Build history of the part. All positions in model axes, mm. Face numbers are marked on the shaded views. A direction names the side the tool comes from. Give positions to 0.01 mm unless a question says otherwise; leave off trailing zeros. Write each loop counter-clockwise with the first axis right and the second up, starting at its lowest first coordinate (ties: lowest second). Pieces come first, ordered by that corner, then holes. Notation, with made-up numbers: (76, 85) -> (116, 85) arc R29 ccw to (116, 113) -> close; hole circle Ø8 at (-21.5, -29.75). An arc over 180 degrees is marked (long way). Put each result on its own line as item: value.
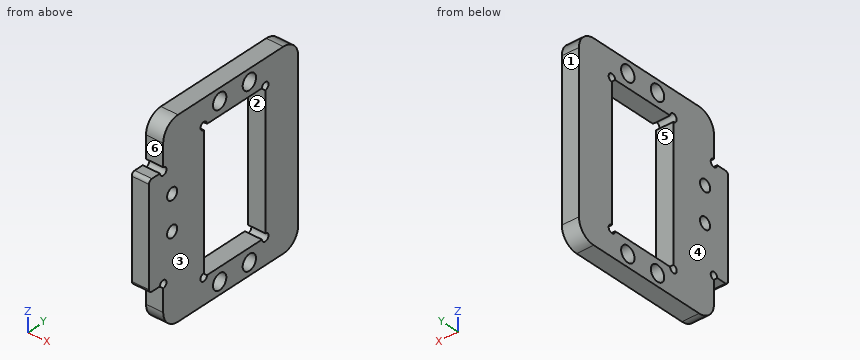
from build123d import *

# Parameters (mm, degrees)
SKETCH_1_W                   = 55
SKETCH_1_H                   = 45.45
SKETCH_1_W_2                 = 40.2
SKETCH_1_H_2                 = 20.7
EXTRUDE_1_DEPTH              = 5
SKETCH_2_W                   = 30
SKETCH_2_H                   = 4.8
EXTRUDE_2_DEPTH              = 5
FILLET_1_R                   = 5
SKETCH_3_R                   = 1.1
CUT_EXTRUDE_1_DEPTH          = 5
FILLET_2_R                   = 1
HOLE_WIZARD_M3_1_D           = 3.4
M4_CLEARANCE_HOLE1_OUTLINE_R = 2.25
M4_CLEARANCE_HOLE1_DEPTH     = 5


# Read off the part's stored shape, not the designer's step: M4 Clearance Hole1
with BuildPart() as part:
    # 草图1 → 凸台-拉伸1 (new body)
    with BuildSketch(Plane(origin=(0, 0, 0), x_dir=(0, 0, -1), z_dir=(1, 0, 0))):
        with Locations((27.5, 22.725)):
            Rectangle(SKETCH_1_W, SKETCH_1_H)
        with Locations((27.5, 24)):
            Rectangle(SKETCH_1_W_2, SKETCH_1_H_2, mode=Mode.SUBTRACT)
    extrude(amount=EXTRUDE_1_DEPTH)

    # 草图2 → 凸台-拉伸2 (add)
    with BuildSketch(Plane(origin=(5, 0, 0), x_dir=(0, 0, -1), z_dir=(1, 0, 0))):
        with Locations((27.5, -2.4)):
            Rectangle(SKETCH_2_W, SKETCH_2_H)
    extrude(amount=-EXTRUDE_2_DEPTH)

    # 圆角1
    fillet_1_edges = [part.edges().sort_by_distance(p)[0] for p in [
        (2.5, 45.45, 0),
        (2.5, 45.45, -55),
        (2.5, 0, -55),
        (2.5, 0, 0),
    ]]
    fillet(fillet_1_edges, radius=FILLET_1_R)

    # 草图3 → 切除-拉伸1 (cut)
    with BuildSketch(Plane(origin=(5, 0, 0), x_dir=(0, 0, -1), z_dir=(1, 0, 0))):
        with Locations((12.5, 0)):
            Circle(SKETCH_3_R)
        with Locations((42.5, 0)):
            Circle(SKETCH_3_R)
        with Locations((7.4, 13.65)):
            Circle(SKETCH_3_R)
        with Locations((7.4, 34.35)):
            Circle(SKETCH_3_R)
        with Locations((47.6, 34.35)):
            Circle(SKETCH_3_R)
        with Locations((47.6, 13.65)):
            Circle(SKETCH_3_R)
    extrude(amount=-CUT_EXTRUDE_1_DEPTH, mode=Mode.SUBTRACT)

    # 圆角2
    fillet_2_edges = [part.edges().sort_by_distance(p)[0] for p in [
        (2.5, -4.8, -42.5),
        (2.5, -4.8, -12.5),
    ]]
    fillet(fillet_2_edges, radius=FILLET_2_R)

    # M3 间隙孔1 (through all)
    with Locations(Plane.ZY):
        with Locations((-20, 3), (-30, 3)):
            Hole(HOLE_WIZARD_M3_1_D / 2)

    # M4 Clearance Hole1 outline → M4 Clearance Hole1 (cut)
    with BuildSketch(Plane.YZ):
        with Locations((29, -3.5)):
            Circle(M4_CLEARANCE_HOLE1_OUTLINE_R)
        with Locations((19, -51.5)):
            Circle(M4_CLEARANCE_HOLE1_OUTLINE_R)
        with Locations((19, -3.5)):
            Circle(M4_CLEARANCE_HOLE1_OUTLINE_R)
        with Locations((29, -51.5)):
            Circle(M4_CLEARANCE_HOLE1_OUTLINE_R)
    extrude(amount=M4_CLEARANCE_HOLE1_DEPTH, mode=Mode.SUBTRACT)


solid = part.part
1) Pin check, flat tips, straight feed: pin 1 (1.5 mm diameter, centred on x = 2, z = -48.5, fed in from -Y); pin 2 (1.8 mm diameter, centred on y = 0, z = -12.5, fed in from -X); pin 3 (2 mm diameter, centred on x = 2, y = -2.5, fed in from -Z). Stop position of each tip, or through.
Filled sheet:
pin 1: y = 0
pin 2: through
pin 3: z = -42.5
2) Slice it at C-C (x = 4.3). Give the number of separate pieces and of enclosed holes in the cut face, plus the area to 3 significant figures.
Filled sheet:
separate pieces: 1
enclosed holes: 7
area: 1,690 mm2
3) Slice it at D-D (y = 3). Write the cut outline in (x, z), plus the area to 3 significant figures.
Filled sheet:
outline: (0, -54.58) -> (5, -54.58) -> (5, -31.7) -> (0, -31.7) -> close; (0, -28.3) -> (5, -28.3) -> (5, -21.7) -> (0, -21.7) -> close; (0, -18.3) -> (5, -18.3) -> (5, -0.42) -> (0, -0.42) -> close
area: 237 mm2
4) Tool access for the marked faces 4, 5 and 6: list every direction of +Z, -Z, +X, -X, +Y, -Y with a clear straight run to the whole face (end or side of a thin tool).
Filled sheet:
face 4: +Z, -Z, -X, +Y, -Y
face 5: +X, -X
face 6: +Z, +X, -X, -Y
5) Wall check: L1, parallel to Y at x = 2.3, z = -30; L2, parallel to Z at x = 1, y = 23.5; L3, parallel to Y at x = 1.15, z = -32.5. Give the ranges that are in metal, low to high.
Filled sheet:
L1: -4.8 to 1.3, 4.7 to 13.65, 34.35 to 45.45
L2: -55 to -47.6, -7.4 to 0
L3: -4.8 to 13.65, 34.35 to 45.45
6) Slice it at B-B (y = 29). Write the cut outline in (x, z), plus the area to 3 significant figures.
Filled sheet:
outline: (0, -55) -> (5, -55) -> (5, -53.75) -> (0, -53.75) -> close; (0, -49.25) -> (5, -49.25) -> (5, -47.6) -> (0, -47.6) -> close; (0, -7.4) -> (5, -7.4) -> (5, -5.75) -> (0, -5.75) -> close; (0, -1.25) -> (5, -1.25) -> (5, 0) -> (0, 0) -> close
area: 29.0 mm2
7) Slice it at A-A (z = -23). Write the cut outline in (x, y).
Filled sheet:
outline: (0, -4.8) -> (5, -4.8) -> (5, 13.65) -> (0, 13.65) -> close; (0, 34.35) -> (5, 34.35) -> (5, 45.45) -> (0, 45.45) -> close
8) Pull direction Y, two halves, no side cores. Call the marked faces 1, 2 and 3: released by +Y, released by -Y, zero draft, split by the parting line, or undercut.
Filled sheet:
face 1: released by +Y
face 2: undercut
face 3: zero draft
